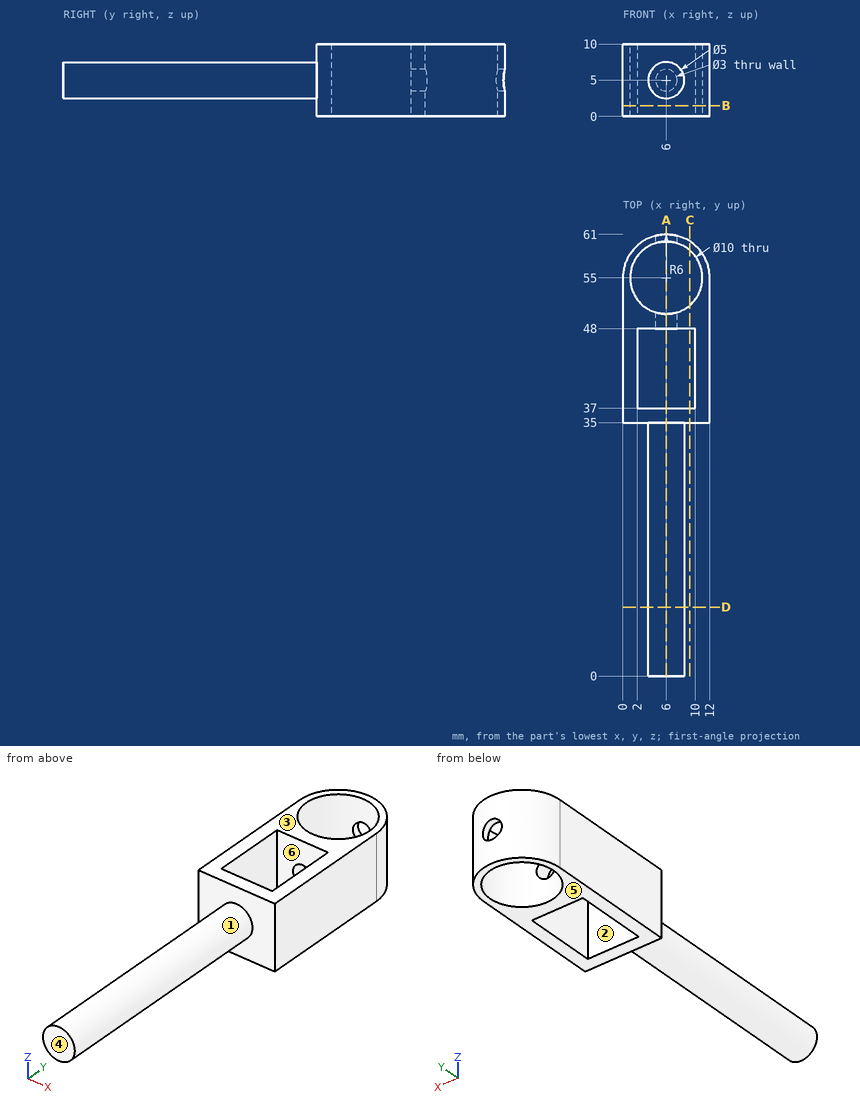
Check sheet for the drawn part. Datum: minimum x, y, z corner. Units: mm. A direction names the side the tool comes from. Coordinates: 2 decimals unless noted, no trailing zeros. Loops run counter-clockwise (first coordinate to the right, second up) from the corner with the lowest first, then second, coordinate; pieces in that order, holes last. Notation, with made-up numbers: (82, 37.25) - (91, 37.25) arc R13 ccw to (91, 41.25) - close; hole circle Ø2 at (58, -26). An arc over 180 degrees is marked (long way). Put each result on its own line as item: value.
Item 1: Draft check along Y on the marked faces 4, 5 and 6. Enter one of: pulls with the +Y half, pulls with the -Y half, needs draft (parallel to the pull), parting line crosses it, or undercut.
Conclusion:
face 4: pulls with the -Y half
face 5: needs draft
face 6: undercut
Item 2: Section check C-C (x = 9.25). Enter the section's corners in (y, z), then the cut area to 3 significant figures.
Conclusion:
outline: (35, 0) - (37, 0) - (37, 10) - (35, 10) - close; (48, 0) - (51.2, 0) - (51.2, 10) - (48, 10) - close; (58.8, 0) - (60.04, 0) - (60.04, 10) - (58.8, 10) - close
area: 64.4 mm2
Item 3: Scan lines: line 1 along Y through (x, z) = (2.75, 1.5); line 2 along Z through (x, y) = (6, 49.1); line 3 along Y through (x, z) = (4.25, 7.5). Record each from-to range of solid material in increasing order.
Conclusion:
line 1: y = 35 to 37, 48 to 51.2, 58.8 to 60.04
line 2: z = 0 to 3.5, 6.5 to 10
line 3: y = 35 to 37, 48 to 50.32, 59.68 to 60.74
Item 4: Section check B-B (z = 1.5). Enter the section's corners in (x, y).
Conclusion:
outline: (0, 35) - (12, 35) - (12, 55) arc R6 ccw to (0, 55) - close; hole circle Ø10 at (6, 55); hole (2, 37) - (10, 37) - (10, 48) - (2, 48) - close
Item 5: Section check D-D (y = 9.5). Enter the section's corners in (x, z), then the cut area to 3 significant figures.
Conclusion:
outline: circle Ø5 at (6, 5)
area: 19.6 mm2
Item 6: Gauge pin test, flat ends, axial feed: pin 1 Ø3 at (x, z) = (1, 4) entering from +Y; pin 2 Ø1.8 at (x, z) = (6, 5) entering from +Y; pin 3 Ø1 at (x, z) = (9, 3) entering from -Y. Record the tip position at first contact, or that the pin passes through.
Conclusion:
pin 1: stops at y = 59.87
pin 2: stops at y = 37
pin 3: stops at y = 35
Item 7: Section check A-A (x = 6). Enter the section's corners in (y, z).
Conclusion:
outline: (0, 2.5) - (35, 2.5) - (35, 0) - (37, 0) - (37, 10) - (35, 10) - (35, 7.5) - (0, 7.5) - close; (48, 0) - (50, 0) - (50, 3.5) - (48, 3.5) - close; (48, 6.5) - (50, 6.5) - (50, 10) - (48, 10) - close; (60, 0) - (61, 0) - (61, 3.5) - (60, 3.5) - close; (60, 6.5) - (61, 6.5) - (61, 10) - (60, 10) - close
Item 8: Set-up check for the marked faces 1, 2 and 3: record each of +Z, -Z, +X, -X, +Y, -Y from which the full face is reachable in a straight line by a thin tool's end or side.
Conclusion:
face 1: -Y
face 2: +Z, -Z
face 3: +Z, +X, -X, +Y, -Y
